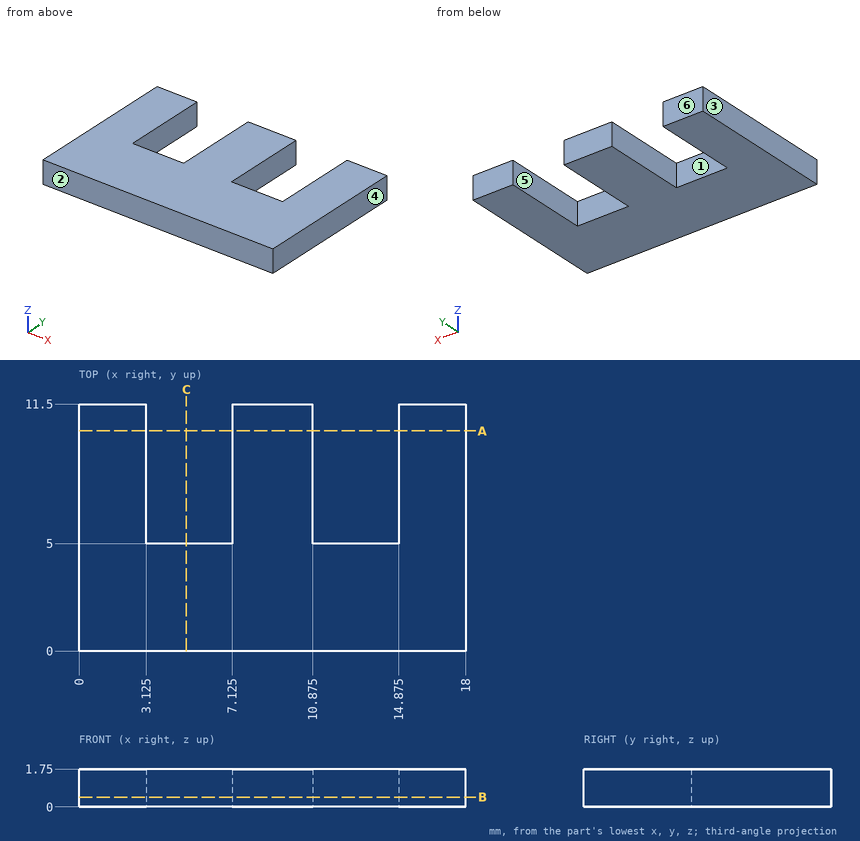
Check sheet for the drawn part. Datum: minimum x, y, z corner. Units: mm. A direction names the side the tool comes from. Coordinates: 2 decimals unless noted, no trailing zeros. Loops run counter-clockwise (first coordinate to the right, second up) from the corner with the lowest first, then second, coordinate; pieces in that order, holes last. Notation, with made-up numbers: (25.25, -23) -> (54.25, -23) arc R23 cw to (54.25, -10) -> close; hole circle Ø6 at (39, 0.25). An arc over 180 degrees is marked (long way). Answer in a Markdown table with one row per item.
1. Sectioned sample at A-A, the plane y = 10.25. Record the boundary of the cut face in (x, z) (3 decimals), then the cut area to 3 significant figures.
Check values:
| item | result |
|---|---|
| outline | (0, 0) -> (3.125, 0) -> (3.125, 1.75) -> (0, 1.75) -> close; (7.125, 0) -> (10.875, 0) -> (10.875, 1.75) -> (7.125, 1.75) -> close; (14.875, 0) -> (18, 0) -> (18, 1.75) -> (14.875, 1.75) -> close |
| area | 17.5 mm2 |
2. Access from +Z, -Z, +X, -X, +Y, -Y to the whole of each face (thin tool, end or side, straight path). Record for the marked faces 5 and 6.
Check values:
| item | result |
|---|---|
| face 5 | +Z, -Z, +Y |
| face 6 | +Z, -Z, +X, -X, +Y |
3. Go/stop test with a flat-tipped pin: pin 1 (0.5 mm diameter, centred on x = 12, z = 0.5, fed in from +Y). Record where the tip stops, or that it passes through.
Check values:
| item | result |
|---|---|
| pin 1 | stops at y = 5 |
4. Material ranges on line 1 along X through (y, z) = (10, 1.45) (3 decimals); line 2 along Y through (x, z) = (12.75, 1.4), recorded low to high. Write a range as [from, to].
Check values:
| item | result |
|---|---|
| line 1 | x = [0, 3.125], [7.125, 10.875], [14.875, 18] |
| line 2 | y = [0, 5] |
5. Sectioned sample at C-C, the plane x = 5. Record the boundary of the cut face in (y, z).
Check values:
| item | result |
|---|---|
| outline | (0, 0) -> (5, 0) -> (5, 1.75) -> (0, 1.75) -> close |
6. Sectioned sample at B-B, the plane z = 0.45. Record the boundary of the cut face in (x, y) (3 decimals).
Check values:
| item | result |
|---|---|
| outline | (0, 0) -> (18, 0) -> (18, 11.5) -> (14.875, 11.5) -> (14.875, 5) -> (10.875, 5) -> (10.875, 11.5) -> (7.125, 11.5) -> (7.125, 5) -> (3.125, 5) -> (3.125, 11.5) -> (0, 11.5) -> close |
7. Release check for a two-part mould opening along X. For the marked faces 1, 2, 3 and 4 record: released by +X, released by -X, zero draft, split by the parting line, or undercut.
Check values:
| item | result |
|---|---|
| face 1 | undercut |
| face 2 | zero draft |
| face 3 | released by -X |
| face 4 | released by +X |
